from build123d import *

# Parameters (mm, degrees)
SALIENTE_EXTRUIR1_DEPTH = 7.5
SALIENTE_EXTRUIR2_DEPTH = 7.5
CROQUIS3_W              = 7.5
CROQUIS3_H              = 7.5
SALIENTE_EXTRUIR3_DEPTH = 30
SALIENTE_EXTRUIR4_DEPTH = 7.5
CROQUIS5_W              = 7.5
CROQUIS5_H              = 7.5
SALIENTE_EXTRUIR5_DEPTH = 37.5
CORTAR_EXTRUIR1_REACH   = 19.2
CROQUIS7_R              = 1.6
CORTAR_EXTRUIR2_DEPTH   = 4.5
CORTAR_EXTRUIR3_REACH   = 7
CROQUIS9_R              = 1.6
CORTAR_EXTRUIR4_DEPTH   = 3
CORTAR_EXTRUIR5_REACH   = 14.7
CROQUIS11_R             = 1.05
CORTAR_EXTRUIR6_DEPTH   = 1.8
CORTAR_EXTRUIR7_REACH   = 79
CROQUIS13_R             = 1.6
CORTAR_EXTRUIR8_DEPTH   = 3
CORTAR_EXTRUIR9_REACH   = 79
CROQUIS16_R             = 1.6
CORTAR_EXTRUIR10_DEPTH  = 3


with BuildPart() as part:
    # Croquis1 → Saliente-Extruir1 (new body)
    with BuildSketch(Plane.XY):
        Polygon((0, 0), (7.5, 0), (7.5, 4.5), (32.7, 4.5), (32.7, 3.5), (35.7, 3.5), (35.7, 9), (33.7, 9), (33.7, 12.2), (53.9, 12.2), (53.9, 10.2), (64.1, 0), (77, 0), (77, 7.5), (67.6, 7.5), (57.9, 17.2), (29.7, 17.2), (21.5, 9), (7.5, 9), (7.5, 7.5), (0, 7.5), align=None)
    extrude(amount=SALIENTE_EXTRUIR1_DEPTH)

    # Croquis2 → Saliente-Extruir2 (add)
    with BuildSketch(Plane.XY.offset(7.5)):
        Polygon((0, 7.5), (7.5, 7.5), (7.5, 9), (35.7, 9), (35.7, 7.5), (35.7, 3.5), (32.7, 3.5), (32.7, 4.5), (7.5, 4.5), (7.5, 0), (0, 0), align=None)
    extrude(amount=SALIENTE_EXTRUIR2_DEPTH)

    # Croquis3 → Saliente-Extruir3 (add)
    with BuildSketch(Plane.XY.offset(15)):
        with Locations((3.75, 3.75)):
            Rectangle(CROQUIS3_W, CROQUIS3_H)
    extrude(amount=SALIENTE_EXTRUIR3_DEPTH)

    # Croquis4 → Saliente-Extruir4 (add)
    with BuildSketch(Plane(origin=(0, 7.5, 0), x_dir=(1, 0, 0), z_dir=(0, 1, 0))):
        Polygon((67.6, -7.5), (69.5, -10.790896534), (69.5, -7.5), align=None)
    extrude(amount=-SALIENTE_EXTRUIR4_DEPTH)

    # Croquis5 → Saliente-Extruir5 (add)
    with BuildSketch(Plane.XY.offset(7.5)):
        with Locations((73.25, 3.75)):
            Rectangle(CROQUIS5_W, CROQUIS5_H)
    extrude(amount=SALIENTE_EXTRUIR5_DEPTH)

    # Croquis7 → Cortar-Extruir1 (cut, up to next)
    with BuildSketch(Plane.XZ, mode=Mode.PRIVATE) as cortar_extruir1_sk1:
        with Locations((73.25, 5)):
            Circle(CROQUIS7_R)
    cortar_extruir1_tool1 = extrude(cortar_extruir1_sk1.sketch, amount=-CORTAR_EXTRUIR1_REACH, mode=Mode.PRIVATE) & part.part
    add(cortar_extruir1_tool1.solids().sort_by_distance((73.25, 0, 5))[0], mode=Mode.SUBTRACT)
    # Croquis7 → Cortar-Extruir1 (cut, up to next)
    with BuildSketch(Plane.XZ, mode=Mode.PRIVATE) as cortar_extruir1_sk2:
        with Locations((73.25, 40)):
            Circle(CROQUIS7_R)
    cortar_extruir1_tool2 = extrude(cortar_extruir1_sk2.sketch, amount=-CORTAR_EXTRUIR1_REACH, mode=Mode.PRIVATE) & part.part
    add(cortar_extruir1_tool2.solids().sort_by_distance((73.25, 0, 40))[0], mode=Mode.SUBTRACT)
    # Croquis7 → Cortar-Extruir1 (cut, up to next)
    with BuildSketch(Plane.XZ, mode=Mode.PRIVATE) as cortar_extruir1_sk3:
        with Locations((3.75, 5)):
            Circle(CROQUIS7_R)
    cortar_extruir1_tool3 = extrude(cortar_extruir1_sk3.sketch, amount=-CORTAR_EXTRUIR1_REACH, mode=Mode.PRIVATE) & part.part
    add(cortar_extruir1_tool3.solids().sort_by_distance((3.75, 0, 5))[0], mode=Mode.SUBTRACT)
    # Croquis7 → Cortar-Extruir1 (cut, up to next)
    with BuildSketch(Plane.XZ, mode=Mode.PRIVATE) as cortar_extruir1_sk4:
        with Locations((3.75, 40)):
            Circle(CROQUIS7_R)
    cortar_extruir1_tool4 = extrude(cortar_extruir1_sk4.sketch, amount=-CORTAR_EXTRUIR1_REACH, mode=Mode.PRIVATE) & part.part
    add(cortar_extruir1_tool4.solids().sort_by_distance((3.75, 0, 40))[0], mode=Mode.SUBTRACT)

    # Croquis8 → Cortar-Extruir2 (cut)
    with BuildSketch(Plane(origin=(0, 9, 0), x_dir=(1, 0, 0), z_dir=(0, 1, 0))):
        Polygon((0.9, -3.354551733), (0.9, -6.645448267), (3.75, -8.290896534), (6.6, -6.645448267), (6.6, -3.354551733), (3.75, -1.709103466), align=None)
        Polygon((0.9, -38.354551733), (0.9, -41.645448267), (3.75, -43.290896534), (6.6, -41.645448267), (6.6, -38.354551733), (3.75, -36.709103466), align=None)
        Polygon((70.4, -38.354551733), (70.4, -41.645448267), (73.25, -43.290896534), (76.1, -41.645448267), (76.1, -38.354551733), (73.25, -36.709103466), align=None)
        Polygon((70.4, -3.354551733), (70.4, -6.645448267), (73.25, -8.290896534), (76.1, -6.645448267), (76.1, -3.354551733), (73.25, -1.709103466), align=None)
    extrude(amount=-CORTAR_EXTRUIR2_DEPTH, mode=Mode.SUBTRACT)

    # Croquis9 → Cortar-Extruir3 (cut, up to next)
    with BuildSketch(Plane.XZ.offset(-12.2), mode=Mode.PRIVATE) as cortar_extruir3_sk1:
        with Locations((51.6, 3.75)):
            Circle(CROQUIS9_R)
    cortar_extruir3_tool1 = extrude(cortar_extruir3_sk1.sketch, amount=-CORTAR_EXTRUIR3_REACH, mode=Mode.PRIVATE) & part.part
    add(cortar_extruir3_tool1.solids().sort_by_distance((51.6, 12.2, 3.75))[0], mode=Mode.SUBTRACT)

    # Croquis10 → Cortar-Extruir4 (cut)
    with BuildSketch(Plane(origin=(0, 17.2, 0), x_dir=(1, 0, 0), z_dir=(0, 1, 0))):
        Polygon((49.954551733, -0.9), (48.309103466, -3.75), (49.954551733, -6.6), (53.245448267, -6.6), (54.890896534, -3.75), (53.245448267, -0.9), align=None)
    extrude(amount=-CORTAR_EXTRUIR4_DEPTH, mode=Mode.SUBTRACT)

    # Croquis11 → Cortar-Extruir5 (cut, up to next)
    with BuildSketch(Plane.XZ.offset(-4.5), mode=Mode.PRIVATE) as cortar_extruir5_sk1:
        with Locations((30.6, 10)):
            Circle(CROQUIS11_R)
    cortar_extruir5_tool1 = extrude(cortar_extruir5_sk1.sketch, amount=-CORTAR_EXTRUIR5_REACH, mode=Mode.PRIVATE) & part.part
    add(cortar_extruir5_tool1.solids().sort_by_distance((30.6, 4.5, 10))[0], mode=Mode.SUBTRACT)
    # Croquis11 → Cortar-Extruir5 (cut, up to next)
    with BuildSketch(Plane.XZ.offset(-4.5), mode=Mode.PRIVATE) as cortar_extruir5_sk2:
        with Locations((9.6, 10)):
            Circle(CROQUIS11_R)
    cortar_extruir5_tool2 = extrude(cortar_extruir5_sk2.sketch, amount=-CORTAR_EXTRUIR5_REACH, mode=Mode.PRIVATE) & part.part
    add(cortar_extruir5_tool2.solids().sort_by_distance((9.6, 4.5, 10))[0], mode=Mode.SUBTRACT)

    # Croquis12 → Cortar-Extruir6 (cut)
    with BuildSketch(Plane(origin=(0, 9, 0), x_dir=(1, 0, 0), z_dir=(0, 1, 0))):
        Polygon((8.358696921, -12.15), (10.841303079, -12.15), (12.082606158, -10), (10.841303079, -7.85), (8.358696921, -7.85), (7.117393842, -10), align=None)
        Polygon((28.117393842, -10), (29.358696921, -12.15), (31.841303079, -12.15), (33.082606158, -10), (31.841303079, -7.85), (29.358696921, -7.85), align=None)
    extrude(amount=-CORTAR_EXTRUIR6_DEPTH, mode=Mode.SUBTRACT)

    # Croquis13 → Cortar-Extruir7 (cut, up to next)
    with BuildSketch(Plane.ZY, mode=Mode.PRIVATE) as cortar_extruir7_sk1:
        with Locations((22.5, 3.75)):
            Circle(CROQUIS13_R)
    cortar_extruir7_tool1 = extrude(cortar_extruir7_sk1.sketch, amount=-CORTAR_EXTRUIR7_REACH, mode=Mode.PRIVATE) & part.part
    add(cortar_extruir7_tool1.solids().sort_by_distance((0, 3.75, 22.5))[0], mode=Mode.SUBTRACT)

    # Croquis15 → Cortar-Extruir8 (cut)
    with BuildSketch(Plane(origin=(7.5, 0, 0), x_dir=(0, 0, -1), z_dir=(1, 0, 0))):
        Polygon((-24.145448267, 0.9), (-20.854551733, 0.9), (-19.209103466, 3.75), (-20.854551733, 6.6), (-24.145448267, 6.6), (-25.790896534, 3.75), align=None)
    extrude(amount=-CORTAR_EXTRUIR8_DEPTH, mode=Mode.SUBTRACT)

    # Croquis16 → Cortar-Extruir9 (cut, up to next)
    with BuildSketch(Plane(origin=(77, 0, 0), x_dir=(0, 0, -1), z_dir=(1, 0, 0)), mode=Mode.PRIVATE) as cortar_extruir9_sk1:
        with Locations((-22.5, 3.75)):
            Circle(CROQUIS16_R)
    cortar_extruir9_tool1 = extrude(cortar_extruir9_sk1.sketch, amount=-CORTAR_EXTRUIR9_REACH, mode=Mode.PRIVATE) & part.part
    add(cortar_extruir9_tool1.solids().sort_by_distance((77, 3.75, 22.5))[0], mode=Mode.SUBTRACT)

    # Croquis17 → Cortar-Extruir10 (cut)
    with BuildSketch(Plane.ZY.offset(-69.5)):
        Polygon((20.854551733, 0.9), (24.145448267, 0.9), (25.790896534, 3.75), (24.145448267, 6.6), (20.854551733, 6.6), (19.209103466, 3.75), align=None)
    extrude(amount=-CORTAR_EXTRUIR10_DEPTH, mode=Mode.SUBTRACT)


solid = part.part
Input: part model. Units: mm. Frame: model coordinates. A direction names the side the tool comes from. Give positions to 0.01 mm unless a question says otherwise; leave off trailing zeros. Loops run counter-clockwise (first coordinate to the right, second up) from the corner with the lowest first, then second, coordinate; pieces in that order, holes last. Notation, with made-up numbers: (-8.75, 0) -> (44.25, 0) arc R16 ccw to (44.25, 29) -> close; hole circle Ø5 at (70.25, 50). An arc over 180 degrees is marked (long way). Answer as a JSON object with one key per item and string values. Group by question number.
Item 1: Cut plane C-C, the plane y = 15.25. Return the cut outline in (x, z).
Item 2: Reachability of faces 1 (the flat face through (6.021, 2.345, 24.98)), 2 (the flat face through (4, 7.5, 22)), 3 (the flat face through (32, 7.2, 10)) from +Z, -Z, +X, -X, +Y, -Y: full face, straight path, thin tool, end or side. Return the list, or none.
Item 3: Cut plane B-B, the plane x = 9.6. Return the cut outline in (y, z), and give its area (3 significant figures).
Item 4: Pin query (flat end, axial travel): P1, Ø1.5, axis at x = 52, y = 16, coming from the +Z side; P2, Ø3, axis at x = 3.75, z = 5, coming from the +Y side; P3, Ø1.5, axis at x = 11.5, y = 5, coming from the +Z side; P4, Ø1.5, axis at x = 71, z = 23, coming from the +Y side. Return the tip coordinate at first contact, or that it passes through.
Item 5: Cut plane D-D, the plane z = 40. Return the cut outline in (x, y), and give its area (3 significant figures).
Item 6: Cut plane A-A, the plane z = 35. Return the cut outline in (x, y), and give its area (4 significant figures).
Item 7: Pull-direction query (Z, two-part tool) for faces 4 (the flat face through (68.537, 3.802, 9.122)), 5 (the flat face through (69.5, 4, 28)), 6 (the flat face through (71, 6.6, 23)); classes: released by +Z, released by -Z, zero draft, split by the parting line, or undercut.
Item 8: Line query: probe 1 along X at (y, z) = (7, 39.5); probe 2 along Z at (x, y) = (3.75, 3.55); probe 3 along X at (y, z) = (5, 26.5). Output: solid intervals per line, ascending.
Checks:
{
 "1": {"outline": "(27.75, 0) -> (59.85, 0) -> (59.85, 7.5) -> (27.75, 7.5) -> close; hole (48.31, 3.75) -> (49.95, 0.9) -> (53.25, 0.9) -> (54.89, 3.75) -> (53.25, 6.6) -> (49.95, 6.6) -> close"},
 "2": {"face 1": "none", "face 2": "+Z, -Z, -X, +Y", "face 3": "+Y"},
 "3": {"outline": "(4.5, 0) -> (9, 0) -> (9, 7.85) -> (7.2, 7.85) -> (7.2, 8.95) -> (4.5, 8.95) -> close; (4.5, 11.05) -> (7.2, 11.05) -> (7.2, 12.15) -> (9, 12.15) -> (9, 15) -> (4.5, 15) -> close", "area": "54.1 mm²"},
 "4": {"P1": "stops at z = 7.5", "P2": "passes through", "P3": "stops at z = 15", "P4": "stops at y = 7.5"},
 "5": {"outline": "(0, 0) -> (2.15, 0) -> (2.15, 4.5) -> (0.9, 4.5) -> (0.9, 7.5) -> (0, 7.5) -> close; (5.35, 0) -> (7.5, 0) -> (7.5, 7.5) -> (6.6, 7.5) -> (6.6, 4.5) -> (5.35, 4.5) -> close; (69.5, 0) -> (71.65, 0) -> (71.65, 4.5) -> (70.4, 4.5) -> (70.4, 7.5) -> (69.5, 7.5) -> close; (74.85, 0) -> (77, 0) -> (77, 7.5) -> (76.1, 7.5) -> (76.1, 4.5) -> (74.85, 4.5) -> close", "area": "49.5 mm²"},
 "6": {"outline": "(0, 0) -> (7.5, 0) -> (7.5, 7.5) -> (0, 7.5) -> close; (69.5, 0) -> (77, 0) -> (77, 7.5) -> (69.5, 7.5) -> close", "area": "112.5 mm²"},
 "7": {"face 4": "released by +Z", "face 5": "zero draft", "face 6": "undercut"},
 "8": {"probe 1": "x = 0 to 0.9, 6.6 to 7.5, 69.5 to 70.4, 76.1 to 77", "probe 2": "z = 0 to 3.4, 6.6 to 20.91, 24.09 to 38.4, 41.6 to 45", "probe 3": "x = 0 to 7.5, 69.5 to 77"}
}
